Design review of the part built by this model. Coordinates are the model's own, in mm. A direction names the side the tool comes from. Round coordinates to 2 decimals unless told otherwise and drop trailing zeros. Loops run counter-clockwise (first coordinate to the right, second up) from the corner with the lowest first, then second, coordinate; pieces in that order, holes last. Notation, with made-up numbers: (73.5, 27.5) - (78.5, 27.5) arc R33 cw to (78.5, 64.5) - close; hole circle Ø2 at (86, 67.5). An arc over 180 degrees is marked (long way). Use one line per item in the form item = value. Start each with the question number.
(1) For pin 1 (3 mm diameter, centred on y = 83.5, z = 17.5, fed in from -X), flat-tipped, find the tip position at first contact; note if it passes through.
(2) The part is to be moulded in two halves that separate along Z. For faces 1 (the flat face through (-12, 95, 13)), 2 (the cylindrical face through (-3, 94, 22)), 3 (the flat face through (0.4, 59.4, 0)), say which applies: released by +Z, released by -Z, zero draft, split by the parting line, or undercut.
(3) We need section C-C, the plane z = 4.88. Give the number of separate pieces and of enclosed holes in the cut face, then the cut area to 3 significant figures.
(4) Wall thickness on probe 1 along X at (y, z) = (46.5, 2.25); probe 2 along Y at (x, z) = (-8.75, 12.25); probe 3 along Y at (x, z) = (1.25, 23.25): over which ranges is each line inside the solid? List them lowest first. Write a range as [from, to].
(5) Machinability: for faces 4 (the flat face through (0, 45, 13)), 5 (the cylindrical face through (1.5, 89, 22.2)), 6 (the flat face through (-13, 94, 6.35)), which of the approach directions +Z, -Z, +X, -X, +Y, -Y give a long, thin tool a straight path to every point of the face, cutting with its end or side? Answer none if there is none.
(6) We need section A-A, the plane x = -17.5. Write out the cut boundary in (y, z), then the cut area to 3 significant figures.
(7) We need section D-D, the plane z = 11.75. Write out the cut boundary in (x, y), then the cut area to 3 significant figures.
(8) We need section B-B, the plane y = 45. Write out the cut boundary in (x, z), then the cut area to 3 significant figures.
from build123d import *

# Parameters (mm, degrees)
BOSS_EXTRUDE1_DEPTH = 27
CUT_EXTRUDE1_DEPTH  = 104.218215447
CUT_EXTRUDE2_DEPTH  = 103.386522551
FILLET1_R           = 3
FILLET2_R           = 3


with BuildPart() as part:
    # Sketch1 → Boss-Extrude1 (new body)
    with BuildSketch(Plane.XY):
        Polygon((0, 0), (3, 0), (3, 95), (-27, 95), (-27, 92), (0, 92), align=None)
    extrude(amount=BOSS_EXTRUDE1_DEPTH)

    # Sketch6 → Cut-Extrude1 (cut, through all)
    with BuildSketch(Plane(origin=(3, 0, 0), x_dir=(0, 0, -1), z_dir=(1, 0, 0))):
        with BuildLine():
            Line((-20.07, 86.95), (-20.07, 5.05))
            ThreePointArc((-20.07, 5.05), (-22.12, 3), (-24.17, 5.05))
            Line((-24.17, 5.05), (-24.17, 86.95))
            ThreePointArc((-24.17, 86.95), (-22.12, 89), (-20.07, 86.95))
        make_face()
        with BuildLine():
            Line((-2.83, 86.95), (-2.83, 5.05))
            ThreePointArc((-2.83, 5.05), (-4.88, 3), (-6.93, 5.05))
            Line((-6.93, 5.05), (-6.93, 86.95))
            ThreePointArc((-6.93, 86.95), (-4.88, 89), (-2.83, 86.95))
        make_face()
    extrude(amount=-CUT_EXTRUDE1_DEPTH, mode=Mode.SUBTRACT)

    # Sketch7 → Cut-Extrude2 (cut, through all)
    with BuildSketch(Plane(origin=(0, 95, 0), x_dir=(1, 0, 0), z_dir=(0, 1, 0))):
        with BuildLine():
            Line((-21.95, -3.65), (-4.35, -3.65))
            ThreePointArc((-4.35, -3.65), (-3, -5), (-4.35, -6.35))
            Line((-4.35, -6.35), (-21.95, -6.35))
            ThreePointArc((-21.95, -6.35), (-23.3, -5), (-21.95, -3.65))
        make_face()
        with BuildLine():
            Line((-21.95, -20.65), (-4.35, -20.65))
            ThreePointArc((-4.35, -20.65), (-3, -22), (-4.35, -23.35))
            Line((-4.35, -23.35), (-21.95, -23.35))
            ThreePointArc((-21.95, -23.35), (-23.3, -22), (-21.95, -20.65))
        make_face()
    extrude(amount=-CUT_EXTRUDE2_DEPTH, mode=Mode.SUBTRACT)

    # Fillet1
    fillet1_edges = [part.edges().sort_by_distance(p)[0] for p in [
        (0, 92, 13.5),
    ]]
    fillet(fillet1_edges, radius=FILLET1_R - 0.0001)  # a hair under: the kernel refuses the full size

    # Fillet2
    fillet2_edges = [part.edges().sort_by_distance(p)[0] for p in [
        (-27, 93.5, 27),
        (-27, 93.5, 0),
        (1.5, 0, 0),
        (1.5, 0, 27),
    ]]
    fillet(fillet2_edges, radius=FILLET2_R)


solid = part.part
Data:
q1.pin_1 = 0
q2.face_1 = zero draft
q2.face_2 = undercut
q2.face_3 = released by -Z
q3.separate_pieces = 3
q3.enclosed_holes = 0
q3.area = 49.1 mm^2
q4.probe_1 = [0, 3]
q4.probe_2 = [92, 95]
q4.probe_3 = [0, 3.34], [88.66, 95]
q5.face_4 = +Z, -Z, -X, -Y
q5.face_5 = +X, -X
q5.face_6 = +Y, -Y
q6.outline = (92, 0) - (95, 0) - (95, 3.65) - (92, 3.65) - close; (92, 6.35) - (95, 6.35) - (95, 20.65) - (92, 20.65) - close; (92, 23.35) - (95, 23.35) - (95, 27) - (92, 27) - close
q6.area = 64.8 mm^2
q7.outline = (-27, 92) - (-3, 92) arc R3 cw to (0, 89) - (0, 0) - (3, 0) - (3, 95) - (-27, 95) - close
q7.area = 368 mm^2
q8.outline = (0, 0) - (3, 0) - (3, 2.83) - (0, 2.83) - close; (0, 6.93) - (3, 6.93) - (3, 20.07) - (0, 20.07) - close; (0, 24.17) - (3, 24.17) - (3, 27) - (0, 27) - close
q8.area = 56.4 mm^2
